```python
from build123d import *

# Parameters (mm, degrees)
EXTRUDE1_DEPTH = 65
FILLET1_R      = 2


with BuildPart() as part:
    # Sketch1 → Extrude1 (new body)
    with BuildSketch(Plane(origin=(0, 0, 0), x_dir=(1, 0, 0), z_dir=(0, 1, 0))):
        with BuildLine():
            Line((-15.155444566, 8.75), (2.344555434, 39.060889132))
            ThreePointArc((2.344555434, 39.060889132), (8.75, 45.466333699), (17.5, 47.810889132))
            Line((17.5, 47.810889132), (87.5, 47.810889132))
            ThreePointArc((87.5, 47.810889132), (96.25, 45.466333699), (102.655444566, 39.060889132))
            Line((102.655444566, 39.060889132), (120.155444566, 8.75))
            ThreePointArc((120.155444566, 8.75), (122.5, 0), (120.155444566, -8.75))
            Line((120.155444566, -8.75), (102.655444566, -39.060889132))
            ThreePointArc((102.655444566, -39.060889132), (96.25, -45.466333699), (87.5, -47.810889132))
            Line((87.5, -47.810889132), (17.5, -47.810889132))
            ThreePointArc((17.5, -47.810889132), (8.75, -45.466333699), (2.344555434, -39.060889132))
            Line((2.344555434, -39.060889132), (-15.155444566, -8.75))
            ThreePointArc((-15.155444566, -8.75), (-17.5, 0), (-15.155444566, 8.75))
        make_face()
    extrude(amount=EXTRUDE1_DEPTH)

    # Fillet1
    fillet1_edges = [part.edges().sort_by_distance(p)[0] for p in [
        (8.75, 65, 45.466333699),
        (-6.405444566, 0, -23.905444566),
        (8.75, 0, -45.466333699),
        (52.5, 0, -47.810889132),
        (96.25, 0, -45.466333699),
        (111.405444566, 0, -23.905444566),
        (122.5, 0, 0),
        (52.5, 65, 47.810889132),
        (111.405444566, 0, 23.905444566),
        (96.25, 0, 45.466333699),
        (52.5, 0, 47.810889132),
        (8.75, 0, 45.466333699),
        (-6.405444566, 0, 23.905444566),
        (-17.5, 0, 0),
        (96.25, 65, 45.466333699),
        (111.405444566, 65, 23.905444566),
        (122.5, 65, 0),
        (111.405444566, 65, -23.905444566),
        (96.25, 65, -45.466333699),
        (52.5, 65, -47.810889132),
        (8.75, 65, -45.466333699),
        (-6.405444566, 65, -23.905444566),
        (-17.5, 65, 0),
        (-6.405444566, 65, 23.905444566),
    ]]
    fillet(fillet1_edges, radius=FILLET1_R)


solid = part.part
```
Read the model definition and answer for the solid it produces. Units are mm, in the model's axes. Round coordinates to 2 decimals unless told otherwise and drop trailing zeros. Loops run counter-clockwise (first coordinate to the right, second up) from the corner with the lowest first, then second, coordinate; pieces in that order, holes last. Notation, with made-up numbers: (13, 20.5) -> (38, 20.5) arc R18 ccw to (38, 50.5) -> close; hole circle Ø8 at (62.25, -6.75). An arc over 180 degrees is marked (long way). One line per item, written item: value.
1) Flat-ended cylindrical pins translate along their axes: P1, Ø6, axis at y = 45, z = 11, coming from the +X side; P2, Ø6, axis at y = 57, z = 18.5, coming from the +X side; P3, Ø12, axis at y = 55, z = -22.5, coming from the -X side. Find the tip coordinate at first contact, or state that the pin passes through.
Answer list:
P1: stops at x = 120.56
P2: stops at x = 116.26
P3: stops at x = -10.68
2) A cutting plane is placed at A-A (y = 31.5). Determine the outline of the cut face in (x, z).
Answer list:
outline: (-15.16, -8.75) -> (2.34, -39.06) arc R17.5 ccw to (17.5, -47.81) -> (87.5, -47.81) arc R17.5 ccw to (102.66, -39.06) -> (120.16, -8.75) arc R17.5 ccw to (120.16, 8.75) -> (102.66, 39.06) arc R17.5 ccw to (87.5, 47.81) -> (17.5, 47.81) arc R17.5 ccw to (2.34, 39.06) -> (-15.16, 8.75) arc R17.5 ccw to start
3) Consider L1, parallel to X at y = 13.5, z = 17; L2, parallel to Z at x = 92, y = 6.5; L3, parallel to X at y = 12, z = -6. Determine where each line is inside the solid, lowest interval first. Write a range as [from, to].
Answer list:
L1: x = [-10.39, 115.39]
L2: z = [-47.22, 47.22]
L3: x = [-16.44, 121.44]
